Autodesk Inventor part; units mm, degrees
ref_plane "YZ Plane" through (0, 0, 0) normal (1, 0, 0) x (0, 1, 0)
ref_plane "XZ Plane" through (0, 0, 0) normal (0, 1, 0) x (-1, 0, 0)
ref_plane "XY Plane" through (0, 0, 0) normal (0, 0, 1) x (1, 0, 0)
ref_plane "Work Plane1" through (0, 0, 0) normal (0, 0, 1) x (1, 0, 0)
sketch "Sketch1" plane through (0, 0, 0) normal (0, 0, 1) x (1, 0, 0)
  line L0 (-192, 0) -> (-192, -43) construction
  line L1 (-192, -43) -> (0, -43) construction
  line L2 (-192, 0) -> (0, 0) construction
  line L3 (-153.9875, -0.508) -> (-153.9875, -42.492)
  line L4 (-153.9875, -42.492) -> (-191.492, -42.492)
  line L5 (-191.492, -42.492) -> (-191.492, -0.508)
  line L6 (-191.492, -0.508) -> (-153.9875, -0.508)
  circle A0 centre (-168, -21.5) radius 7.975 construction
  circle A1 centre (-168, -21.5) radius 8.89
  circle A2 centre (-184, -37.5) radius 2 construction
  circle A3 centre (-160, -37.5) radius 2 construction
  circle A4 centre (-160, -5.5) radius 2 construction
  circle A5 centre (-184, -37.5) radius 2.1844
  circle A6 centre (-160, -37.5) radius 2.1844
  circle A7 centre (-160, -5.5) radius 2.1844
extrude "Extrusion1" add sketch "Sketch1" along normal blind 4.064
sketch "Sketch2" plane through (0, 0, 4.064) normal (0, 0, 1) x (1, 0, 0)
  arc A0 (-188.6973, -7.9203) -> (-188.6973, -10.181) centre (-188.5276, -9.0507) ccw construction
  arc A1 (-173.6259, -10.181) -> (-173.6259, -7.9203) centre (-173.7956, -9.0507) ccw construction
  circle A2 centre (-188.5276, -9.0507) radius 1.3716
  circle A3 centre (-173.7956, -9.0507) radius 1.3716
  point P0 (0, 0)
  dimension "d7" = 2.7432
  dimension "d8" = 2.7432
extrude "Extrusion2" cut sketch "Sketch2" against normal through all
sketch "Sketch4" plane through (0, 0, 4.064) normal (0, 0, 1) x (1, 0, 0)
  circle A0 centre (-188.5276, -9.0507) radius 1.3716 construction
  circle A1 centre (-188.5276, -9.0507) radius 2.794 construction
  circle A2 centre (-173.7956, -9.0507) radius 1.3716 construction
  circle A3 centre (-173.7956, -9.0507) radius 2.794 construction
  line L0 (-188.5276, -11.8447) -> (-190.9473, -10.4477)
  line L1 (-190.9473, -10.4477) -> (-190.9473, -7.6537)
  line L2 (-190.9473, -7.6537) -> (-188.5276, -6.2567)
  line L3 (-188.5276, -6.2567) -> (-186.108, -7.6537)
  line L4 (-186.108, -7.6537) -> (-186.108, -10.4477)
  line L5 (-186.108, -10.4477) -> (-188.5276, -11.8447)
  line L6 (-173.7956, -11.8447) -> (-176.2153, -10.4477)
  line L7 (-176.2153, -10.4477) -> (-176.2153, -7.6537)
  line L8 (-176.2153, -7.6537) -> (-173.7956, -6.2567)
  line L9 (-173.7956, -6.2567) -> (-171.376, -7.6537)
  line L10 (-171.376, -7.6537) -> (-171.376, -10.4477)
  line L11 (-171.376, -10.4477) -> (-173.7956, -11.8447)
  point P0 (0, 0)
  dimension "d15" = 5.588
  dimension "d16" = 5.588
extrude "Extrusion4" cut sketch "Sketch4" against normal blind 2.032
properties part number "BallMountRight"
The model under review builds one solid part; all positions refer to its coordinate system, in mm. A direction names the side the tool comes from. Give positions to 0.01 mm unless a question says otherwise; leave off trailing zeros. Write each loop counter-clockwise with the first axis right and the second up, starting at its lowest first coordinate (ties: lowest second). Pieces come first, ordered by that corner, then holes.
(1) For P1, Ø1.5, axis at x = -173, y = -9.5, coming from the +Z side; P2, Ø4, axis at x = -160, y = -5.5, coming from the -Z side, all flat-tipped, find the tip position at first contact; note any pin that passes through.
(2) The part is to be moulded in two halves that separate along Y. For faces 1 (the flat face through (-172.569, -11.136, 3.062)), 2 (the flat face through (-153.988, -21, 2)), 3 (the flat face through (-172, -42.492, 2)), say which applies: released by +Y, released by -Y, zero draft, split by the parting line, or undercut.
(3) Consider section A-A, the plane x = -168. Give the boundary of the cut face in (y, z).
(4) Consider section C-C, the plane y = -5.5. Give the boundary of the cut face in (x, z), and give its area (3 significant figures).
(5) Consider section D-D, the plane z = 2.7. Give the boundary of the cut face in (x, y), and give its area (3 significant figures).
(6) Consider section B-B, the plane y = -37.5. Give the boundary of the cut face in (x, z).
(7) Tool access review of faces 4 (the flat face through (-177.2, -21.2, 0)), 5 (the flat face through (-175.022, -6.965, 3.062)): name each direction out of +Z, -Z, +X, -X, +Y, -Y from which nothing blocks a thin tool from reaching the whole face with its end or side.
(8) To check wall thickness, follow L1, parallel to X at y = -9, z = 1.85; L2, parallel to Y at x = -175.5, z = 2.25; L3, parallel to Y at x = -160, z = 1.9. State the ranges of each line that lie inside material, in increasing order.
Returned:
1. P1: stops at z = 2.03
1. P2: passes through
2. face 1: undercut
2. face 2: zero draft
2. face 3: released by -Y
3. outline: (-42.49, 0) - (-30.39, 0) - (-30.39, 4.06) - (-42.49, 4.06) - close; (-12.61, 0) - (-0.51, 0) - (-0.51, 4.06) - (-12.61, 4.06) - close
4. outline: (-191.49, 0) - (-162.18, 0) - (-162.18, 4.06) - (-191.49, 4.06) - close; (-157.82, 0) - (-153.99, 0) - (-153.99, 4.06) - (-157.82, 4.06) - close
4. area: 135 mm2
5. outline: (-191.49, -42.49) - (-153.99, -42.49) - (-153.99, -0.51) - (-191.49, -0.51) - close; hole (-190.95, -10.45) - (-188.53, -11.84) - (-186.11, -10.45) - (-186.11, -7.65) - (-188.53, -6.26) - (-190.95, -7.65) - close; hole circle Ø4.37 at (-184, -37.5); hole circle Ø17.78 at (-168, -21.5); hole (-176.22, -10.45) - (-173.8, -11.84) - (-171.38, -10.45) - (-171.38, -7.65) - (-173.8, -6.26) - (-176.22, -7.65) - close; hole circle Ø4.37 at (-160, -37.5); hole circle Ø4.37 at (-160, -5.5)
5. area: 1,240 mm2
6. outline: (-191.49, 0) - (-186.18, 0) - (-186.18, 4.06) - (-191.49, 4.06) - close; (-181.82, 0) - (-162.18, 0) - (-162.18, 4.06) - (-181.82, 4.06) - close; (-157.82, 0) - (-153.99, 0) - (-153.99, 4.06) - (-157.82, 4.06) - close
7. face 4: -Z, +X, -X, +Y, -Y
7. face 5: +Z
8. L1: x = -191.49 to -189.9, -187.16 to -175.17, -172.42 to -153.99
8. L2: y = -42.49 to -26.27, -16.73 to -10.86, -7.24 to -0.51
8. L3: y = -42.49 to -39.68, -35.32 to -25.38, -17.62 to -7.68, -3.32 to -0.51
